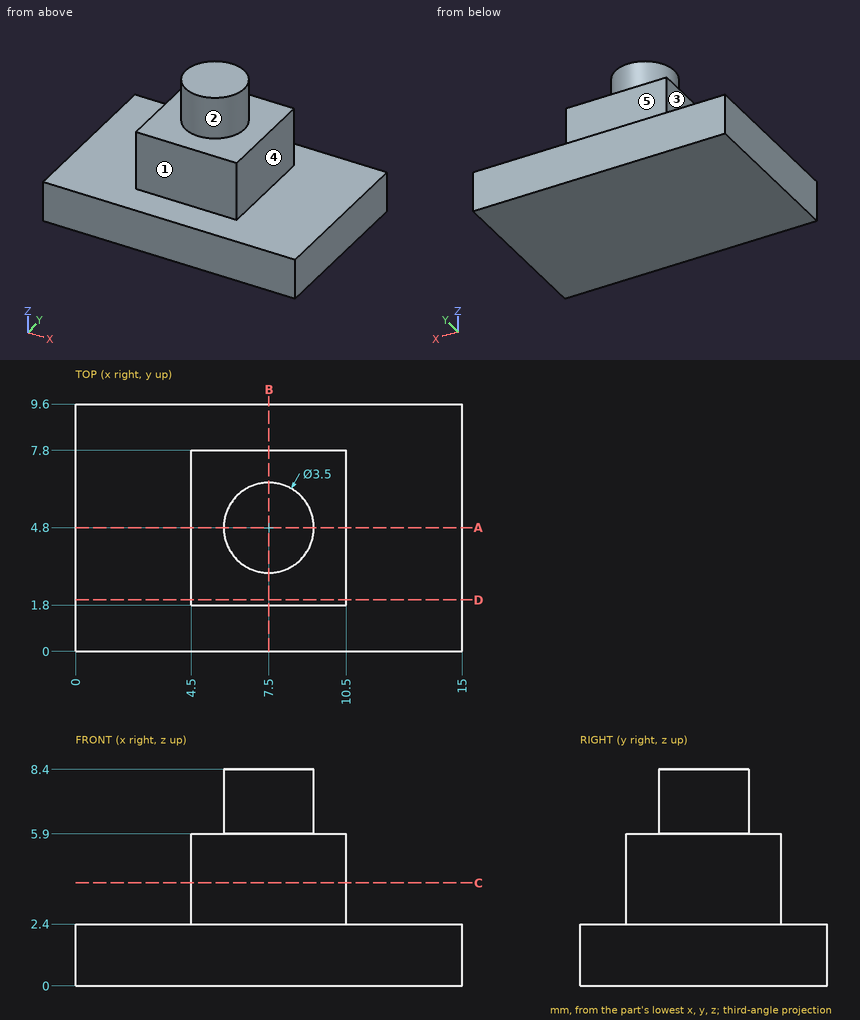
Job drawing, mm, ordinate dimensions from the low corner. One solid piece. A direction names the side the tool comes from. Round coordinates to 2 decimals unless told otherwise and drop trailing zeros. Loops run counter-clockwise (first coordinate to the right, second up) from the corner with the lowest first, then second, coordinate; pieces in that order, holes last. Notation, with made-up numbers: (66.5, 32.25) -> (70.5, 32.25) arc R21 cw to (70.5, 61.25) -> close; hole circle Ø9 at (83.25, 70.5). An arc over 180 degrees is marked (long way). One line per item, written item: value. Start each with the question number.
Q1. Cut at A-A on y = 4.8. List the corners of the cut face in (x, z), plus the area to 4 significant figures.
Q2. Cut at C-C on z = 4. List the corners of the cut face in (x, y), plus the area to 3 significant figures.
Q3. Cut at D-D on y = 2. List the corners of the cut face in (x, z).
Q4. Drop flat-ended pins along their axis: pin 1 Ø1.8 at (y, z) = (5.5, 5) entering from +X; pin 2 Ø3 at (x, z) = (9, 4.5) entering from +Y; pin 3 Ø1.8 at (y, z) = (5, 5) entering from -X. Give the stop position or say it passes through.
Q5. Probe line 1 along Z through (x, y) = (6, 0.75); line 2 along Z through (x, y) = (8.5, 6.75); line 3 along Y through (x, z) = (7.75, 3.25). List the from-to ranges inside material, lowest first.
Q6. 3-axis set-ups, long thin cutter, end or side, ignore diameter. For the marked faces 1, 2, 3, 4 and 5: which of +Z, -Z, +X, -X, +Y, -Y reach the whole face in a straight line?
Q7. Cut at B-B on x = 7.5. List the corners of the cut face in (y, z).
Computed:
1. outline: (0, 0) -> (15, 0) -> (15, 2.4) -> (10.5, 2.4) -> (10.5, 5.9) -> (9.25, 5.9) -> (9.25, 8.4) -> (5.75, 8.4) -> (5.75, 5.9) -> (4.5, 5.9) -> (4.5, 2.4) -> (0, 2.4) -> close
1. area: 65.75 mm²
2. outline: (4.5, 1.8) -> (10.5, 1.8) -> (10.5, 7.8) -> (4.5, 7.8) -> close
2. area: 36.0 mm²
3. outline: (0, 0) -> (15, 0) -> (15, 2.4) -> (10.5, 2.4) -> (10.5, 5.9) -> (4.5, 5.9) -> (4.5, 2.4) -> (0, 2.4) -> close
4. pin 1: x = 10.5
4. pin 2: y = 7.8
4. pin 3: x = 4.5
5. line 1: 0 to 2.4
5. line 2: 0 to 5.9
5. line 3: 1.8 to 7.8
6. face 1: +Z, +X, -X, -Y
6. face 2: +Z
6. face 3: +Z, -X, +Y, -Y
6. face 4: +Z, +X, +Y, -Y
6. face 5: +Z, +X, -X, +Y
7. outline: (0, 0) -> (9.6, 0) -> (9.6, 2.4) -> (7.8, 2.4) -> (7.8, 5.9) -> (6.55, 5.9) -> (6.55, 8.4) -> (3.05, 8.4) -> (3.05, 5.9) -> (1.8, 5.9) -> (1.8, 2.4) -> (0, 2.4) -> close
